Read the model definition and answer for the solid it produces. Units are mm, in the model's axes. A direction names the side the tool comes from. Coordinates: 2 decimals unless noted, no trailing zeros. Order: outer loops, then holes, each group sorted by start corner. A loop starts at its lowest first (then second) coordinate and runs counter-clockwise, first axis right, second up. Notation, with made-up numbers: (8, -31.75) - (14, -31.75) arc R34 cw to (14, 4.25) - close; hole circle Ø3 at (-19, -4.5). An arc over 180 degrees is marked (long way). Use one line per item in the form item = value.
```python
from build123d import *

# Parameters (mm, degrees)
SKETCH1_W           = 14.732
SKETCH1_H           = 46.99
BOSS_EXTRUDE1_DEPTH = 12.7
SKETCH2_W           = 16.51
SKETCH2_H           = 19.304
CUT_EXTRUDE1_DEPTH  = 15.732
CUT_EXTRUDE2_REACH  = 48.99
SKETCH3_R           = 2.286
SKETCH4_W           = 7.747
SKETCH4_H           = 25.4
CUT_EXTRUDE3_DEPTH  = 20.955
SKETCH5_R           = 3.175
CUT_EXTRUDE4_DEPTH  = 15.732


with BuildPart() as part:
    # Sketch1 → Boss-Extrude1 (new body, symmetric)
    with BuildSketch(Plane(origin=(0, 0, 0), x_dir=(1, 0, 0), z_dir=(0, 1, 0))):
        Rectangle(SKETCH1_W, SKETCH1_H)
    extrude(amount=BOSS_EXTRUDE1_DEPTH, both=True)

    # Sketch2 → Cut-Extrude1 (cut, through all)
    with BuildSketch(Plane(origin=(7.366, 0, 0), x_dir=(0, 0, -1), z_dir=(1, 0, 0))):
        with Locations((-9.652, 3.048)):
            Rectangle(SKETCH2_W, SKETCH2_H)
    extrude(amount=-CUT_EXTRUDE1_DEPTH, mode=Mode.SUBTRACT)

    # Sketch3 → Cut-Extrude2 (cut, up to next)
    with BuildSketch(Plane.XY.offset(23.495), mode=Mode.PRIVATE) as cut_extrude2_sk1:
        with Locations((1.016, 0)):
            Circle(SKETCH3_R)
    cut_extrude2_tool1 = extrude(cut_extrude2_sk1.sketch, amount=-CUT_EXTRUDE2_REACH, mode=Mode.PRIVATE) & part.part
    add(cut_extrude2_tool1.solids().sort_by_distance((1.016, 0, 23.495))[0], mode=Mode.SUBTRACT)

    # Sketch4 → Cut-Extrude3 (cut)
    with BuildSketch(Plane(origin=(0, 0, -23.495), x_dir=(-1, 0, 0), z_dir=(0, 0, -1))):
        with Locations((-3.4925, 0)):
            Rectangle(SKETCH4_W, SKETCH4_H)
    extrude(amount=-CUT_EXTRUDE3_DEPTH, mode=Mode.SUBTRACT)

    # Sketch5 → Cut-Extrude4 (cut, through all)
    with BuildSketch(Plane.ZY.offset(7.366)):
        with Locations((-15.24, 6.35)):
            Circle(SKETCH5_R)
    extrude(amount=-CUT_EXTRUDE4_DEPTH, mode=Mode.SUBTRACT)


solid = part.part
```
(1) Section B-B, the plane x = -2.25 is taken. Write down the section's boundary in (y, z) (3 decimals).
Answer list:
outline = (-12.7, -23.495) - (12.7, -23.495) - (12.7, 1.397) - (-6.604, 1.397) - (-6.604, 17.907) - (12.7, 17.907) - (12.7, 23.495) - (-12.7, 23.495) - close; hole circle Ø6.35 at (6.35, -15.24)
(2) Section A-A, the plane z = -15.24 is taken. Write down the section's boundary in (x, y) (3 decimals).
Answer list:
outline = (-7.366, -12.7) - (-0.381, -12.7) - (-0.381, 3.175) - (-7.366, 3.175) - close; (-7.366, 9.525) - (-0.381, 9.525) - (-0.381, 12.7) - (-7.366, 12.7) - close
(3) Given pin 1 Ø2 at (y, z) = (2.5, -9) entering from +X; pin 2 Ø6 at (x, y) = (4.5, -5) entering from -Z; pin 3 Ø2 at (x, z) = (-2.5, 12.5) entering from +Y, each flat-ended and moving along its own axis, determine where each tip first touches the part or whether it passes through.
Answer list:
pin_1 = -0.38
pin_2 = -2.54
pin_3 = -6.6
(4) Which of the six approach directions +Z, -Z, +X, -X, +Y, -Y give full straight-line access (tool end or side, diameter ignored) to faces 5 (the flat face through (7.366, -8, 14)), 6 (the flat face through (0, 3, 17.907)), 7 (the flat face through (-0.381, 0, -13))?
Answer list:
face_5 = +Z, -Z, +X, +Y, -Y
face_6 = +X, -X, +Y
face_7 = -Z, +X, +Y, -Y
(5) Section D-D, the plane x = 6 is taken. Write down the section's boundary in (y, z) (3 decimals).
Answer list:
outline = (-12.7, -2.54) - (12.7, -2.54) - (12.7, 1.397) - (-6.604, 1.397) - (-6.604, 17.907) - (12.7, 17.907) - (12.7, 23.495) - (-12.7, 23.495) - close
(6) Straight lines are drawn through the part: L1, parallel to Y at x = -6, z = -15.24 (3 decimals); L2, parallel to Z at x = -5.5, y = -0.5 (3 decimals); L3, parallel to Z at x = 4.25, y = -4.25 (3 decimals). For each, find the intervals that lie inside material, in ascending order.
Answer list:
L1 = -12.7 to 3.175, 9.525 to 12.7
L2 = -23.495 to 1.397, 17.907 to 23.495
L3 = -2.54 to 1.397, 17.907 to 23.495
(7) Section C-C, the plane y = 0 is taken. Write down the section's boundary in (x, z) (3 decimals).
Answer list:
outline = (-7.366, -23.495) - (-0.381, -23.495) - (-0.381, -2.54) - (7.366, -2.54) - (7.366, 1.397) - (-7.366, 1.397) - close; (-7.366, 17.907) - (-1.27, 17.907) - (-1.27, 23.495) - (-7.366, 23.495) - close; (3.302, 17.907) - (7.366, 17.907) - (7.366, 23.495) - (3.302, 23.495) - close
(8) The mould has two halves that part along Y. Classify faces 1 (the flat face through (0, -6.604, 10)), 2 (the flat face through (-2, 0, 23.495)), 3 (the cylindrical face through (-0.8, -1.39, 20.74)), 4 (the cylindrical face through (-3.922, 9.027, -13.533)): +Y half, -Y half, draft (parallel to the pull), parting line (faces both ways), or undercut.
Answer list:
face_1 = +Y half
face_2 = draft
face_3 = undercut
face_4 = undercut
